from build123d import *

# Parameters (mm, degrees)
SWEEP1_PROFILE_R = 12.7
SHELL2_T         = -6.35


with BuildPart() as part:
    # Sweep1: sweep along a path in Sketch1
    with BuildLine(Plane.XY) as sweep1_path:
        Line((38.1, 608.33), (38.1, 25.4))
        ThreePointArc((38.1, 25.4), (30.660512242, 7.439487758), (12.7, 0))
        Line((12.7, 0), (0, 0))
    # Sweep1 profile (on start of the path) → Sweep1 (sweep)
    with BuildSketch(Plane(origin=(38.1, 608.33, 0), x_dir=(-1, 0, 0), z_dir=(0, -1, 0))):
        Circle(SWEEP1_PROFILE_R)
    sweep(path=sweep1_path.line)

    # Shell2
    shell2_openings = [part.faces().sort_by_distance(p)[0] for p in [
        (0, 12.7, 0),
        (25.4, 608.33, 0),
    ]]
    offset(amount=SHELL2_T, openings=shell2_openings, kind=Kind.INTERSECTION)


solid = part.part
Model file for the job. Use its own axes, mm. Give positions to 0.01 mm unless a question says otherwise; leave off trailing zeros. Loops run counter-clockwise (first coordinate to the right, second up) from the corner with the lowest first, then second, coordinate; pieces in that order, holes last. Notation, with made-up numbers: (13.5, 70) -> (32.5, 70) arc R29 cw to (32.5, 109) -> close; hole circle Ø1 at (23.5, -10). An arc over 180 degrees is marked (long way). Use a Markdown table: item, result. Add a question column.
(1) Drop flat-ended pins along their axis: pin 1 Ø3 at (y, z) = (216.5, -3) entering from +X; pin 2 Ø3 at (x, y) = (37.5, 366.5) entering from -Z; pin 3 Ø12 at (x, z) = (41.5, -3.5) entering from -Y; pin 4 Ø4 at (x, y) = (27.5, 269) entering from -Z. Give the stop position or say it passes through.
(2) Slice it at C-C on x = 6. List the corners of the cut face in (y, z), and give its area (3 significant figures).
(3) Wall check: line 1 along Y through (x, z) = (8.5, 0); line 2 along X through (y, z) = (552, 0.5). Give the ranges that are in metal, low to high.
(4) Slice it at B-B on y = 223. List the corners of the cut face in (x, z), and give its area (3 significant figures).
(5) Slice it at A-A on z = 0. List the corners of the cut face in (x, y).
(6) Mould opens along X. For faces 1 (the cylindrical face through (32.043, 312.784, -1.907)), 2 (the cylindrical face through (48.2, 312.8, 7.7)), 3 (the flat face through (0, -6, -3)), 4 (the flat face through (35, 608.33, 6)) say: +X half, -X half, draft (parallel to the pull), parting line (faces both ways), or undercut.
Filled sheet:
| question | item | result |
|---|---|---|
| 1 | pin 1 | x = 50.71 |
| 1 | pin 2 | z = -12.7 |
| 1 | pin 3 | y = -4.78 |
| 1 | pin 4 | z = -9.35 |
| 2 | outline | circle Ø25.4 at (0, 0); hole circle Ø12.7 at (0, 0) |
| 2 | area | 380 mm2 |
| 3 | line 1 | -12.7 to -6.35, 6.35 to 12.7 |
| 3 | line 2 | 25.41 to 31.77, 44.43 to 50.79 |
| 4 | outline | circle Ø25.4 at (38.1, 0); hole circle Ø12.7 at (38.1, 0) |
| 4 | area | 380 mm2 |
| 5 | outline | (0, -12.7) -> (12.7, -12.7) arc R38.1 ccw to (50.8, 25.4) -> (50.8, 608.33) -> (44.45, 608.33) -> (44.45, 25.4) arc R31.75 cw to (12.7, -6.35) -> (0, -6.35) -> close; (0, 6.35) -> (12.7, 6.35) arc R19.05 ccw to (31.75, 25.4) -> (31.75, 608.33) -> (25.4, 608.33) -> (25.4, 25.4) arc R12.7 cw to (12.7, 12.7) -> (0, 12.7) -> close |
| 6 | face 1 | undercut |
| 6 | face 2 | parting line |
| 6 | face 3 | -X half |
| 6 | face 4 | draft |
